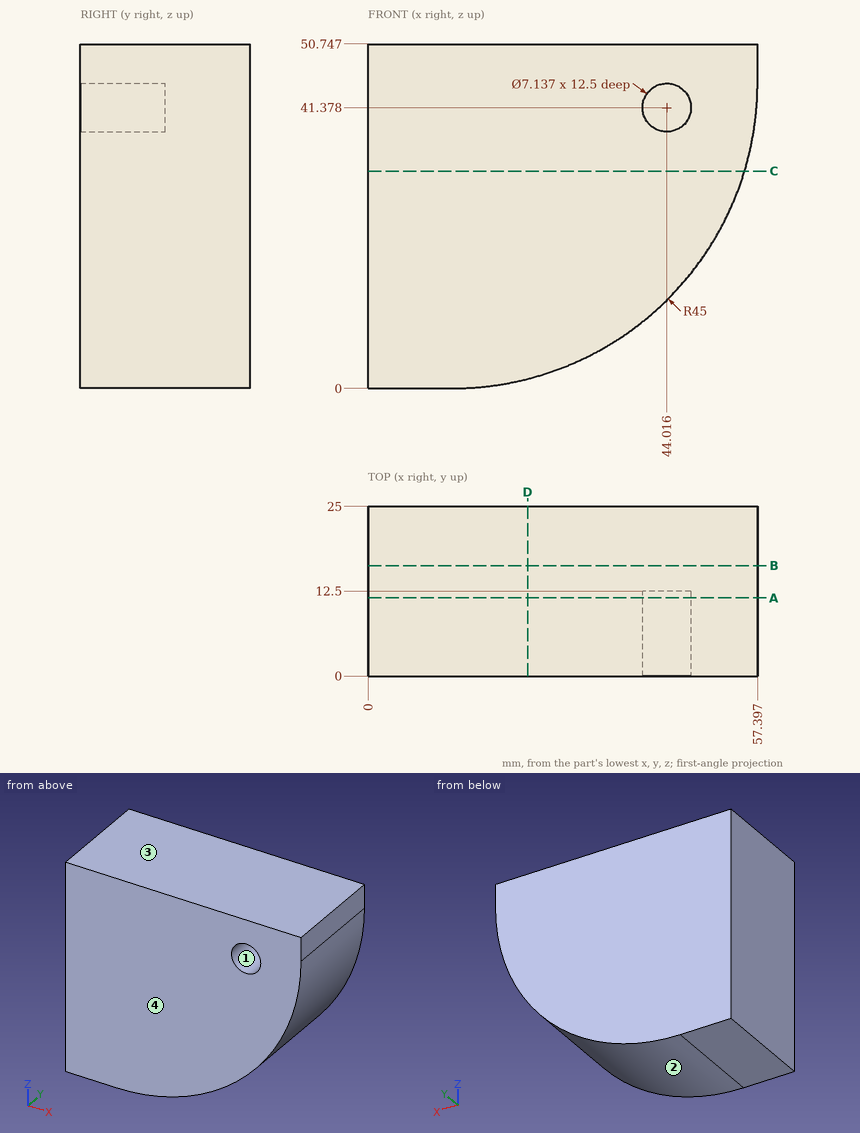
Answer from the drawing. Dimensions are ordinates in mm from the lowest x, y and z of the part. Coordinates: 2 decimals unless noted, no trailing zeros. Write each loop counter-clockwise with the first axis right and the second up, starting at its lowest first coordinate (ties: lowest second). Pieces come first, ordered by that corner, then holes. Notation, with made-up numbers: (72, -4.75) -> (84, -4.75) arc R23 cw to (84, 26.25) -> close; hole circle Ø2 at (81.5, 64). An arc over 180 degrees is marked (long way). One line per question, with ' | ' between items.
1. Section C-C (z = 32) is taken. Determine the outline of the cut face in (x, y).
Verdict:
outline: (0, 0) -> (55.48, 0) -> (55.48, 25) -> (0, 25) -> close
2. Section A-A (y = 11.5) is taken. Determine the outline of the cut face in (x, z) (1 decimal).
Verdict:
outline: (0, 0) -> (12.4, 0) arc R45 ccw to (57.4, 45) -> (57.4, 50.7) -> (0, 50.7) -> close; hole circle Ø7.1 at (44, 41.4)
3. Section B-B (y = 16.25) is taken. Determine the outline of the cut face in (x, z), and give its area (3 significant figures).
Verdict:
outline: (0, 0) -> (12.4, 0) arc R45 ccw to (57.4, 45) -> (57.4, 50.75) -> (0, 50.75) -> close | area: 2,480 mm^2
4. Straight lines are drawn through the part: line 1 (Z direction, x = 43.5, y = 5) (1 decimal); line 2 (Y direction, x = 42.5, z = 38.5); line 3 (Z direction, x = 44, y = 11) (1 decimal). For each, find the intervals that lie inside material, in ascending order.
Verdict:
line 1: z = 12.5 to 37.8, 44.9 to 50.7 | line 2: y = 12.5 to 25 | line 3: z = 13 to 37.8, 44.9 to 50.7
5. For a pull along Z with two mould halves and no side action, classify the marked faces 1, 2, 3 and 4 as released by +Z, released by -Z, zero draft, split by the parting line, or undercut.
Verdict:
face 1: undercut | face 2: released by -Z | face 3: released by +Z | face 4: zero draft
6. Given pin 1 Ø3 at (y, z) = (8.5, 16.5) entering from +X; pin 2 Ø3 at (x, y) = (34.5, 8.5) entering from -Z; pin 3 Ø4 at (y, z) = (17.5, 35) entering from +X, each flat-ended and moving along its own axis, determine where each tip first touches the part or whether it passes through.
Verdict:
pin 1: stops at x = 48.4 | pin 2: stops at z = 4.99 | pin 3: stops at x = 56.68
7. Section D-D (x = 23.5) is taken. Determine the outline of the cut face in (y, z), and give its area (3 significant figures).
Verdict:
outline: (0, 1.39) -> (25, 1.39) -> (25, 50.75) -> (0, 50.75) -> close | area: 1,230 mm^2
